Verification items for the finished model (mm, model axes). Face numbers are marked on the shaded views. A direction names the side the tool comes from. Round coordinates to 2 decimals unless told otherwise and drop trailing zeros. Order: outer loops, then holes, each group sorted by start corner. A loop starts at its lowest first (then second) coordinate and runs counter-clockwise, first axis right, second up. Notation, with made-up numbers: (-0.75, 49) -> (16.25, 49) arc R27 ccw to (16.25, 72) -> close; hole circle Ø11 at (-2.75, -6). An arc over 180 degrees is marked (long way). Return JSON: item names as keys, results as strings. Group by question number.
Item 1: Access from +Z, -Z, +X, -X, +Y, -Y to the whole of each face (thin tool, end or side, straight path). Record for the marked faces 1 and 2.
Item 2: Depth check by flat-ended pin: pin 1 Ø6 at (x, y) = (-2, -1) entering from -Z. Enter the tip coordinate at first touch or a pass-through.
Item 3: Draft check along Z on the marked faces 3, 4 and 5. Enter one of: pulls with the +Z half, pulls with the -Z half, needs draft (parallel to the pull), parting line crosses it, or undercut.
Item 4: Sectioned sample at A-A on z = 10.5. Record the cut outline in (x, y).
Item 5: Sectioned sample at C-C on y = -3.5. Record the cut outline in (x, z), plus the area to 3 significant figures.
Item 6: Sectioned sample at B-B on x = -14. Record the cut outline in (y, z), plus the area to 3 significant figures.
Item 7: Sectioned sample at D-D on y = 1. Record the cut outline in (x, z).
Item 8: Scan lines: probe 1 along X at (y, z) = (-1.5, 7.75); probe 2 along Y at (x, z) = (24.5, 0.6); probe 3 along Z at (x, y) = (-27, 3.75). Record each from-to range of solid material in increasing order. Write a range as from..to.
```python
from build123d import *

# Parameters (mm, degrees)
F0_W      = 60
F0_H      = 12
F1_DEPTH  = 20
F2_W      = 42
F2_H      = 2
F3_DEPTH  = 12.001
F4_DEPTH  = 12.001
F6_D      = 3.3
F6_DEPTH  = 2.001
F8_D      = 3.3
F8_DEPTH  = 2.001
F10_D     = 3.6
F10_DEPTH = 12
F10_TIP   = 1.0815491142
F9_W      = 10
F9_H      = 3.6
F11_DEPTH = 12.5


with BuildPart() as f1:
    # F0 (on Top) → F1 (new body)
    with BuildSketch(Plane.XY):
        Rectangle(F0_W, F0_H)
    extrude(amount=F1_DEPTH)

    # F2 (on face) → F3 (cut, through all)
    with BuildSketch(Plane.XZ.offset(6)):
        Polygon((28, 18), (-28, 18), (-28, 2), (-21, 2), (21, 2), (28, 2), align=None)
        with Locations((0, 1)):
            Rectangle(F2_W, F2_H)
    extrude(amount=-F3_DEPTH, mode=Mode.SUBTRACT)

    # F2 (on face) → F4 (cut, through all)
    with BuildSketch(Plane.XZ.offset(6)):
        Polygon((28, 18), (-28, 18), (-28, 2), (-21, 2), (21, 2), (28, 2), align=None)
        with Locations((0, 1)):
            Rectangle(F2_W, F2_H)
    extrude(amount=-F4_DEPTH, mode=Mode.SUBTRACT)

    # F6 (through all, one way)
    with BuildSketch(Plane.XY.offset(2)):
        with Locations((-24.5, 0)):
            Circle(F6_D / 2)
    extrude(amount=-F6_DEPTH, mode=Mode.SUBTRACT)

    # F8 (through all, one way)
    with BuildSketch(Plane.XY.offset(2)):
        with Locations((24.5, 0)):
            Circle(F8_D / 2)
    extrude(amount=-F8_DEPTH, mode=Mode.SUBTRACT)

    # F10
    with Locations(Plane.XY.offset(20)):
        with Locations((-15, 0), (15, 0), (-25, 0), (25, 0)):
            Hole(F10_D / 2, depth=F10_DEPTH)
            with Locations((0, 0, -(F10_DEPTH + F10_TIP / 2))):  # 118° drill point
                Cone(0, F10_D / 2, F10_TIP, mode=Mode.SUBTRACT)

    # F9 (on face) → F11 (cut, symmetric)
    with BuildSketch(Plane.XY.offset(20)):
        with Locations((-20, 0)):
            Rectangle(F9_W, F9_H)
        with Locations((20, 0)):
            Rectangle(F9_W, F9_H)
    extrude(amount=F11_DEPTH, both=True, mode=Mode.SUBTRACT)


solid = f1.part
```
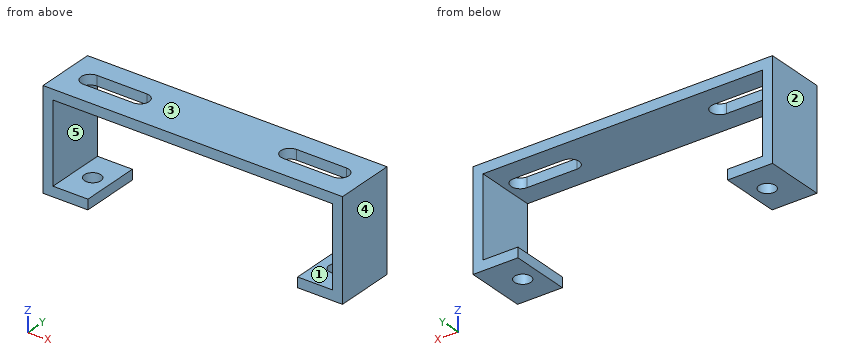
Recorded:
{
 "1": {"face 1": "+Y, -Y", "face 2": "+Z, -Z, -X, +Y, -Y"},
 "2": {"pin 1": "z = 18"},
 "3": {"face 3": "pulls with the +Z half", "face 4": "needs draft", "face 5": "undercut"},
 "4": {"outline": "(-30, -6) -> (-28, -6) -> (-28, 6) -> (-30, 6) -> close; (28, -6) -> (30, -6) -> (30, 6) -> (28, 6) -> close"},
 "5": {"outline": "(-30, 0) -> (-21, 0) -> (-21, 2) -> (-28, 2) -> (-28, 18) -> (28, 18) -> (28, 2) -> (21, 2) -> (21, 0) -> (30, 0) -> (30, 20) -> (-30, 20) -> close", "area": "220 mm²"},
 "6": {"outline": "(-6, 18) -> (-1.5, 18) -> (-1.5, 20) -> (-6, 20) -> close; (1.5, 18) -> (6, 18) -> (6, 20) -> (1.5, 20) -> close", "area": "18.0 mm²"},
 "7": {"outline": "(-30, 0) -> (-25.81, 0) -> (-25.81, 2) -> (-28, 2) -> (-28, 18) -> (-26.5, 18) -> (-26.5, 20) -> (-30, 20) -> close; (-23.19, 0) -> (-21, 0) -> (-21, 2) -> (-23.19, 2) -> close; (-13.5, 18) -> (13.5, 18) -> (13.5, 20) -> (-13.5, 20) -> close; (21, 0) -> (23.19, 0) -> (23.19, 2) -> (21, 2) -> close; (25.81, 0) -> (30, 0) -> (30, 20) -> (26.5, 20) -> (26.5, 18) -> (28, 18) -> (28, 2) -> (25.81, 2) -> close"},
 "8": {"probe 1": "-30..-28, 28..30", "probe 2": "-6..-1.65, 1.65..6", "probe 3": "0..2, 18..20"}
}
